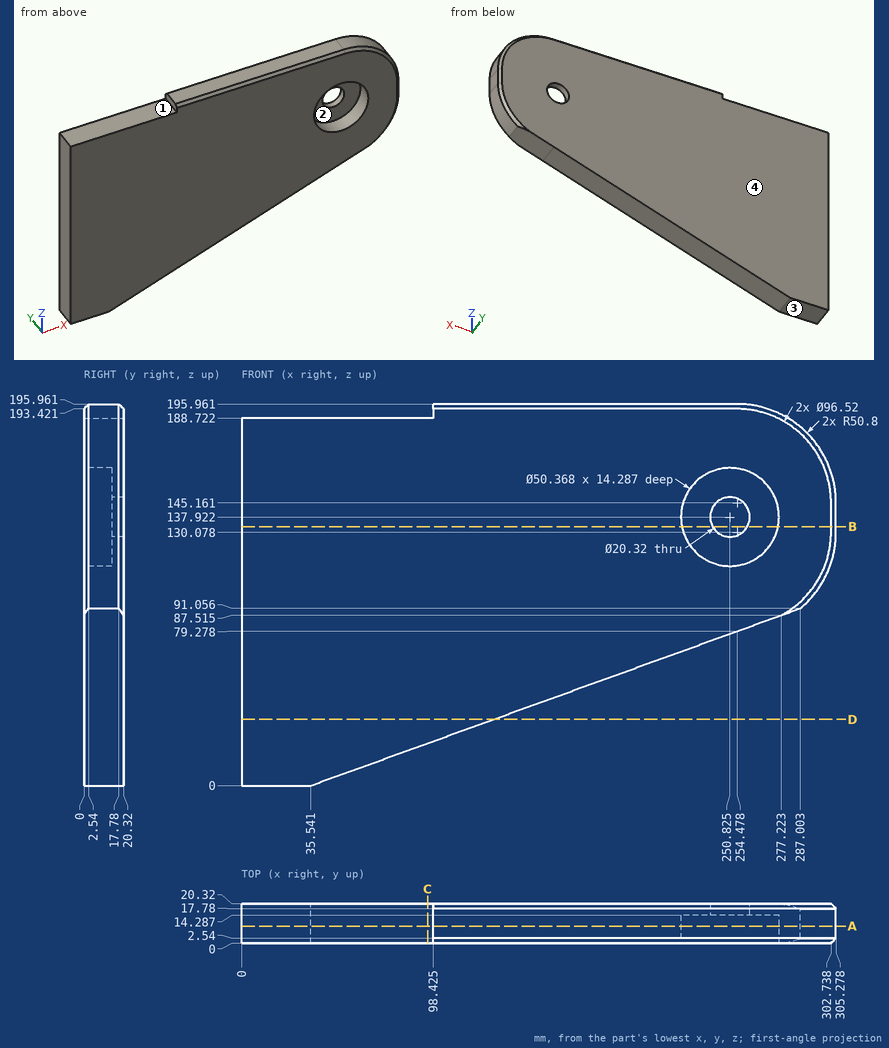
Design review of the part shown in the three views and the two pictorial views. Dimensions are in mm from the part's minimum x, y and z. Give positions to 0.01 mm unless a question says otherwise; leave off trailing zeros. Order: outer loops, then holes, each group sorted by start corner. A loop starts at its lowest first (then second) coordinate and runs counter-clockwise, first axis right, second up. Notation, with made-up numbers: M 74.5,52 L 117.5,52 A6 cw 117.5,58 Z; hole C 46,-6 d7. An arc over 180 degrees is marked long. Answer in a Markdown table with one row per item. Add a question column.
(1) Consider section B-B on z = 133. State the section outline as (x, y) points, and give its area (3 significant figures).
(2) Consider section A-A on y = 8.75. State the section outline as (x, z) points (1 decimal), and give its area (3 significant figures).
(3) Consider section D-D on z = 34. State the section outline as (x, y) points.
(4) Mouldability with a two-part tool opening along Z and no side actions: class the marked faces 1, 2, 3 and 4 as +Z half, -Z half, draft (parallel to the pull), parting line (faces both ways), or undercut.
(5) Consider section C-C on x = 95.5. State the section outline as (y, z) points, and give its area (3 significant figures).
(6) Wall thickness on probe 1 along X at (y, z) = (2.25, 120) (1 decimal); probe 2 along Z at (x, y) = (18.5, 16.5); probe 3 along Z at (x, y) = (263, 5.5) (1 decimal): over which ranges is each line inside the solid? List them lowest first. Write a range as [from, to].
(7) For pin 1 (15 mm diameter, centred on x = 245, z = 137.5, fed in from -Y); pin 2 (8 mm diameter, centred on x = 111.5, y = 3, fed in from -Z); pin 3 (6 mm diameter, centred on y = 9.5, z = 192.5, fed in from -X) (1 decimal), all flat-tipped, find the tip position at first contact; note any pin that passes through.
Evaluation:
| question | item | result |
|---|---|---|
| 1 | outline | M 0,0 L 226.13,0 L 226.13,14.29 L 241.94,14.29 L 241.94,20.32 L 0,20.32 Z; M 259.71,14.29 L 275.52,14.29 L 275.52,0 L 302.74,0 L 305.28,2.54 L 305.28,17.78 L 302.74,20.32 L 259.71,20.32 Z |
| 1 | area | 5,380 mm^2 |
| 2 | outline | M 0,0 L 35.5,0 L 287,91.1 A50.8 ccw 305.3,130.1 L 305.3,145.2 A50.8 ccw 254.5,196 L 98.4,196 L 98.4,188.7 L 0,188.7 Z; hole C 250.8,137.9 d50.4 |
| 2 | area | 43,200 mm^2 |
| 3 | outline | M 0,0 L 129.44,0 L 129.44,20.32 L 0,20.32 Z |
| 4 | face 1 | +Z half |
| 4 | face 2 | undercut |
| 4 | face 3 | -Z half |
| 4 | face 4 | draft |
| 5 | outline | M 0,21.71 L 20.32,21.71 L 20.32,188.72 L 0,188.72 Z |
| 5 | area | 3,390 mm^2 |
| 6 | probe 1 | x = [0, 233.1], [268.5, 304] |
| 6 | probe 2 | z = [0, 188.72] |
| 6 | probe 3 | z = [82.4, 115.9], [160, 195.2] |
| 7 | pin 1 | stops at y = 14.29 |
| 7 | pin 2 | stops at z = 26.06 |
| 7 | pin 3 | stops at x = 98.4 |
